The listing builds one solid part. Answer for the finished solid, in the listing's coordinates (mm). A direction names the side the tool comes from. Give positions to 0.01 mm unless a question says otherwise; leave off trailing zeros. Order: outer loops, then holes, each group sorted by start corner. A loop starts at its lowest first (then second) coordinate and runs counter-clockwise, first axis right, second up. Notation, with made-up numbers: (-4, 70) - (15, 70) arc R18 ccw to (15, 79) - close; hole circle Ø8 at (0.5, -9.5). An arc over 180 degrees is marked (long way). Answer as a JSON object with one key per item and string values. Group by question number.
Q1. A cutting plane is placed at B-B, the plane x = 51. Give the vertices of the cut face in (y, z), and give its area (3 significant figures).
Q2. A cutting plane is placed at C-C, the plane z = 16. Give the vertices of the cut face in (x, y), and give its area (3 significant figures).
Q3. For faces 5 (the face through (55.8, 6, 6)), 6 (the face through (-6, 7, 9.016)), 7 (the face through (-9, 3, 10)), determine the directions among +Z, -Z, +X, -X, +Y, -Y from which every point of the face is accessible in a straight line to the end or side of a thin tool.
Q4. A cutting plane is placed at D-D, the plane x = 29. Give the vertices of the cut face in (y, z), and give its area (3 significant figures).
Q5. Given pin 1 (3.5 mm diameter, centred on y = 8.5, z = 4, fed in from -X); pin 2 (1.2 mm diameter, centred on x = 65, y = 1.5, fed in from -Z); pin 3 (1.7 mm diameter, centred on x = -5, y = 6.5, fed in from +Z); pin 4 (13.5 mm diameter, centred on x = 34.5, z = 18.5, fed in from +Y), each flat-ended and moving along its own axis, determine where each tip first touches the part or whether it passes through.
Q6. A cutting plane is placed at A-A, the plane y = 10.75. Give the vertices of the cut face in (x, z), and give its area (3 significant figures).
Q7. The mould has two halves that part along Y. Classify faces 1 (the face through (48, 7, 9.016)), 2 (the face through (48, 2, 2)), 3 (the face through (48, 12, 4)), 4 (the face through (48.306, 9.264, 4.703)): released by +Y, released by -Y, zero draft, split by the parting line, or undercut.
Q8. Consider line 1 (X direction, y = 6.5, z = 6.25); line 2 (Z direction, x = 52.5, y = 7.25); line 3 (Y direction, x = 0, z = 21). Determine where each line is inside the solid, lowest interval first.
from build123d import *

# Parameters (mm, degrees)
SKETCH_1_W          = 85
SKETCH_1_H          = 26
EXTRUDE_1_DEPTH     = 12
SKETCH_2_W          = 19.106704299
SKETCH_2_H          = 9.017669608
CUT_EXTRUDE_1_DEPTH = 90.693923986
CHAMFER_1_SIZE      = 2.2
CHAMFER_2_SIZE      = 4
SKETCH_3_R          = 1.5
CUT_EXTRUDE_2_DEPTH = 90.693923986
SKETCH_4_W          = 14.2
SKETCH_4_H          = 12
CUT_EXTRUDE_3_DEPTH = 82.215762017


with BuildPart() as part:
    # Эскиз1 → Вытянуть1 (new body)
    with BuildSketch(Plane(origin=(0, 0, 0), x_dir=(1, 0, 0), z_dir=(0, 1, 0))):
        with Locations((33.5, -13)):
            Rectangle(SKETCH_1_W, SKETCH_1_H)
    extrude(amount=EXTRUDE_1_DEPTH)

    # Эскиз2 → Вырез-Вытянуть1 (cut, through all)
    with BuildSketch(Plane(origin=(76, 0, 0), x_dir=(0, 0, -1), z_dir=(1, 0, 0))):
        with Locations((-18.569613205, 8.508834804)):
            Rectangle(SKETCH_2_W, SKETCH_2_H)
    extrude(amount=-CUT_EXTRUDE_1_DEPTH, mode=Mode.SUBTRACT)

    # Фаска1
    chamfer_1_edges = [part.edges().sort_by_distance(p)[0] for p in [
        (33.5, 12, 0),
        (33.5, 12, 9.016261055),
    ]]
    chamfer(chamfer_1_edges, length=CHAMFER_1_SIZE)

    # Фаска2
    chamfer_2_edges = [part.edges().sort_by_distance(p)[0] for p in [
        (33.5, 0, 0),
    ]]
    chamfer(chamfer_2_edges, length=CHAMFER_2_SIZE)

    # Эскиз3 → Вырез-Вытянуть2 (cut, through all)
    with BuildSketch(Plane(origin=(76, 0, 0), x_dir=(0, 0, -1), z_dir=(1, 0, 0))):
        with Locations((-4.508130527, 7.777054312)):
            Circle(SKETCH_3_R)
    extrude(amount=-CUT_EXTRUDE_2_DEPTH, mode=Mode.SUBTRACT)

    # Эскиз4 → Вырез-Вытянуть3 (cut, through all)
    with BuildSketch(Plane(origin=(0, 12, 0), x_dir=(1, 0, 0), z_dir=(0, 1, 0))):
        with Locations((4.1, -6)):
            Rectangle(SKETCH_4_W, SKETCH_4_H)
        with Locations((62.9, -6)):
            Rectangle(SKETCH_4_W, SKETCH_4_H)
        with Locations((33.5, -6)):
            Rectangle(SKETCH_4_W, SKETCH_4_H)
    extrude(amount=-CUT_EXTRUDE_3_DEPTH, mode=Mode.SUBTRACT)


solid = part.part
Reply:
{
 "1": {"outline": "(0, 4) - (4, 0) - (9.8, 0) - (12, 2.2) - (12, 6.82) - (9.8, 9.02) - (4, 9.02) - (4, 26) - (0, 26) - close; hole circle Ø3 at (7.78, 4.51)", "area": "156 mm^2"},
 "2": {"outline": "(-9, 0) - (76, 0) - (76, 4) - (-9, 4) - close", "area": "340 mm^2"},
 "3": {"face 5": "-Z, +Y, -Y", "face 6": "+Z, +X, -X, +Y", "face 7": "+Z, -Z, -X, +Y, -Y"},
 "4": {"outline": "(0, 12) - (4, 12) - (4, 26) - (0, 26) - close", "area": "56.0 mm^2"},
 "5": {"pin 1": "stops at x = -9", "pin 2": "stops at z = 12", "pin 3": "stops at z = 9.02", "pin 4": "stops at y = 4"},
 "6": {"outline": "(-9, 0.95) - (-3, 0.95) - (-3, 8.07) - (-9, 8.07) - close; (11.2, 0.95) - (26.4, 0.95) - (26.4, 8.07) - (11.2, 8.07) - close; (40.6, 0.95) - (55.8, 0.95) - (55.8, 8.07) - (40.6, 8.07) - close; (70, 0.95) - (76, 0.95) - (76, 8.07) - (70, 8.07) - close", "area": "302 mm^2"},
 "7": {"face 1": "zero draft", "face 2": "released by -Y", "face 3": "released by +Y", "face 4": "undercut"},
 "8": {"line 1": "x = -9 to -3, 11.2 to 26.4, 40.6 to 55.8, 70 to 76", "line 2": "z = 0 to 3.1, 5.91 to 9.02", "line 3": "y = 0 to 4"}
}
